```python
from build123d import *

# Parameters (mm, degrees)
F0_R     = 1.651
F1_DEPTH = 15.24
F2_W     = 3.81
F2_H     = 2.733839
F4_R     = 0.719831
F5_DEPTH = 3.811
F6_DEPTH = 3.811


with BuildPart() as f1:
    # F0 (on Top) → F1 (new body)
    with BuildSketch(Plane.XY):
        Circle(F0_R)
    extrude(amount=F1_DEPTH)

    # F2 (on Front) → F3 (revolve)
    with BuildSketch(Plane.XZ):
        with Locations((1.905, 16.606919)):
            Rectangle(F2_W, F2_H)
    revolve(axis=Axis((0, 0, 16.606919), (0, 0, 1)))

    # F4 (on Front) → F5 (cut, through all)
    with BuildSketch(Plane.XZ):
        with Locations((0, 1.905)):
            Circle(F4_R)
    extrude(amount=-F5_DEPTH, mode=Mode.SUBTRACT)

    # F4 (on Front) → F6 (cut, through all)
    with BuildSketch(Plane.XZ):
        with Locations((0, 1.905)):
            Circle(F4_R)
    extrude(amount=F6_DEPTH, mode=Mode.SUBTRACT)


solid = f1.part
```
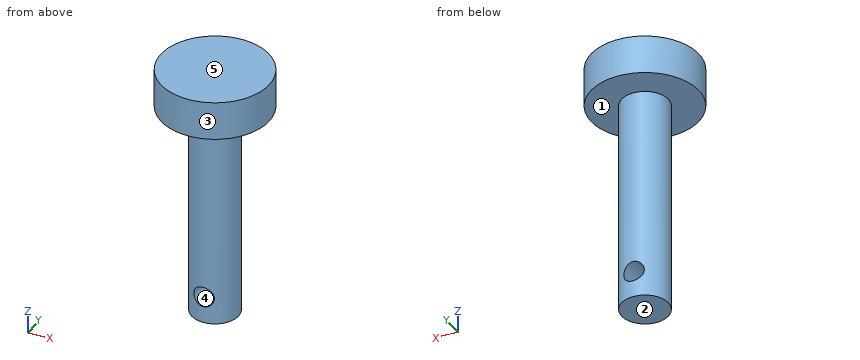
Part model, mm, in its own coordinate system. Face numbers are marked on the shaded views. A direction names the side the tool comes from. Round coordinates to 2 decimals unless told otherwise and drop trailing zeros. Order: outer loops, then holes, each group sorted by start corner. A loop starts at its lowest first (then second) coordinate and runs counter-clockwise, first axis right, second up. Notation, with made-up numbers: M 26,58.25 L 85,58.25 A15 ccw 85,71.25 Z; hole C 27.5,-34.5 d11. An arc over 180 degrees is marked long. Answer in a Markdown table with one row per item. Add a question column.
Q1. Cut at D-D on x = 1. Give the cut face in (y, z), and give its area (3 significant figures).
Q2. Cut at C-C on z = 2.25. Give the cut face in (x, y).
Q3. Cut at B-B on y = 0. Give the cut face in (x, z) (3 decimals), and give its area (3 significant figures).
Q4. Pin check, flat tips, straight feed: pin 1 (2 mm diameter, centred on y = -1, z = 2, fed in from -X); pin 2 (1.5 mm diameter, centred on x = -1.5, z = 3.5, fed in from +Y); pin 3 (1.3 mm diameter, centred on x = 0, z = 1.905, fed in from +Y); pin 4 (1.5 mm diameter, centred on x = 1, y = 3, fed in from -Z). Stop position of each tip, or through.
Q5. Wall check: L1, parallel to Z at x = 0, y = 0.05; L2, parallel to Z at x = 0.25, y = 2; L3, parallel to Y at x = -3, z = 16.5. Give the ranges that are in metal, low to high. Write a range as from..to.
Q6. 3-axis set-ups, long thin cutter, end or side, ignore diameter. For the marked faces 1 and 2: which of +Z, -Z, +X, -X, +Y, -Y reach the whole face in a straight line?
Q7. Mould opens along Z. For the marked faces 3, 4 and 5 say: +Z half, -Z half, draft (parallel to the pull), parting line (faces both ways), or undercut.
Q8. Cut at A-A on x = 0. Give the cut face in (y, z).
Established:
| question | item | result |
|---|---|---|
| 1 | outline | M -3.68,15.24 L -1.31,15.24 L -1.31,0 L 1.31,0 L 1.31,15.24 L 3.68,15.24 L 3.68,17.97 L -3.68,17.97 Z |
| 1 | area | 60.1 mm2 |
| 2 | outline | M -0.63,-1.53 L -0.63,1.53 A1.65 ccw Z; M 0.63,-1.53 A1.65 ccw 0.63,1.53 Z |
| 3 | outline | M -3.81,15.24 L -1.651,15.24 L -1.651,0 L 1.651,0 L 1.651,15.24 L 3.81,15.24 L 3.81,17.974 L -3.81,17.974 Z; hole C 0,1.905 d1.44 |
| 3 | area | 69.5 mm2 |
| 4 | pin 1 | stops at x = -1.65 |
| 4 | pin 2 | stops at y = 1.47 |
| 4 | pin 3 | passes through |
| 4 | pin 4 | stops at z = 15.24 |
| 5 | L1 | z = 0..1.19, 2.62..17.97 |
| 5 | L2 | z = 15.24..17.97 |
| 5 | L3 | y = -2.35..2.35 |
| 6 | face 1 | -Z |
| 6 | face 2 | -Z, +X, -X, +Y, -Y |
| 7 | face 3 | draft |
| 7 | face 4 | undercut |
| 7 | face 5 | +Z half |
| 8 | outline | M -3.81,15.24 L -1.65,15.24 L -1.65,2.62 L 1.65,2.62 L 1.65,15.24 L 3.81,15.24 L 3.81,17.97 L -3.81,17.97 Z; M -1.65,0 L 1.65,0 L 1.65,1.19 L -1.65,1.19 Z |
